Source: three-view drawing plus pictorial views. Frame: mm from the lowest corner of the part. A direction names the side the tool comes from. Give positions to 0.01 mm unless a question says otherwise; leave off trailing zeros. Loops run counter-clockwise (first coordinate to the right, second up) from the corner with the lowest first, then second, coordinate; pieces in that order, holes last.
1. Section C-C, the plane y = 55.5. Output: boundary loops of the cut face in (x, z), then the cut area to 4 significant figures.
2. Section A-A, the plane y = 189. Output: boundary loops of the cut face in (x, z).
3. Material intervals for line 1 along X through (y, z) = (201.75, 40); line 2 along X through (y, z) = (212, 40); line 3 along Z through (x, y) = (155, 203), sorted ascending.
4. Section D-D, the plane z = 71. Output: boundary loops of the cut face in (x, y).
5. Access query for the marked faces 3 and 4. Directions: +Z, -Z, +X, -X, +Y, -Y. A direction counts if a zero-diameter tool reaches every point of the face in a straight line with its end or side. Return the directions, or none.
6. Draft query along X for the marked faces 1 and 2. Return one class per face: +X half, -X half, draft (parallel to the pull), parting line (faces both ways), or undercut.
7. First-contact query: P1, Ø10, axis at x = 212, z = 43, coming from the -Y side; P2, Ø3, axis at x = 108.5, z = 21.5, coming from the -Y side (1 decimal); P3, Ø15, axis at x = 353.5, y = 192, coming from the +Z side; P4, Ø4.5, axis at x = 275, z = 40, coming from the -Y side. Flat tips, straight axial feed; report the tip coordinate or a pass-through.
8. Section B-B, the plane x = 411. Output: boundary loops of the cut face in (y, z).
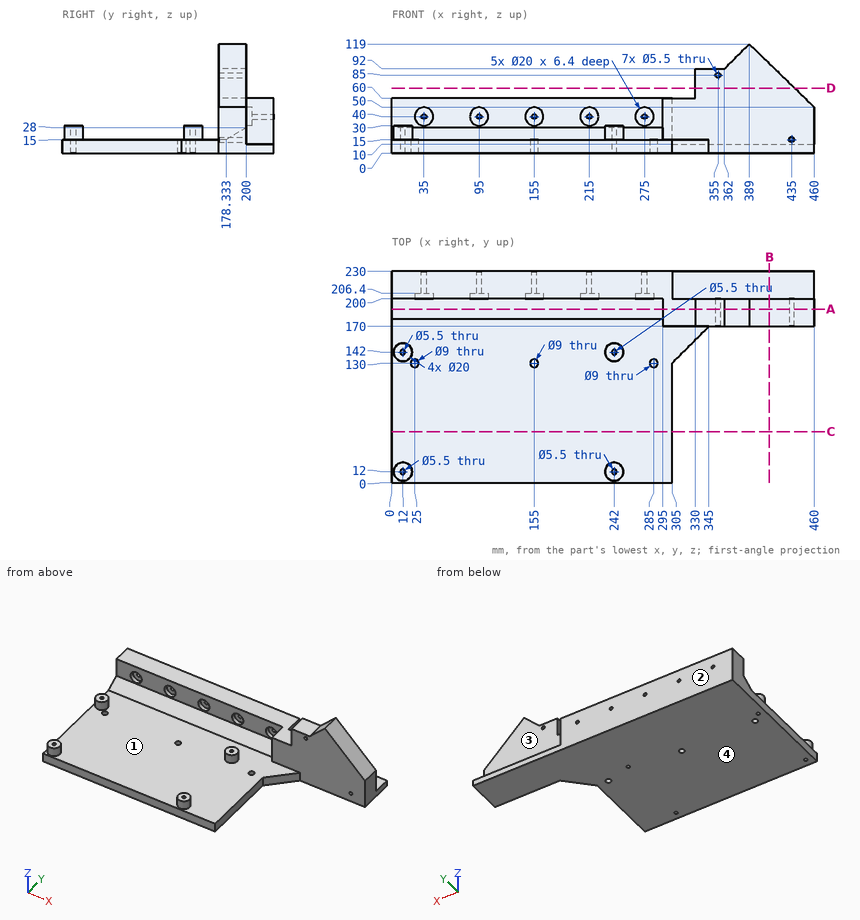
Answers below:
1. outline: (0, 0) - (305, 0) - (305, 15) - (0, 15) - close
1. area: 4,575 mm2
2. outline: (0, 0) - (460, 0) - (460, 50) - (389, 119) - (362, 92) - (330, 92) - (330, 60) - (295, 60) - (295, 21.4) - (0, 21.4) - close; hole circle Ø5.5 at (355, 85); hole circle Ø5.5 at (435, 15)
3. line 1: x = 0 to 25, 45 to 85, 105 to 145, 165 to 205, 225 to 265, 285 to 305
3. line 2: x = 0 to 32.25, 37.75 to 92.25, 97.75 to 152.25, 157.75 to 212.25, 217.75 to 272.25, 277.75 to 305
3. line 3: z = 0 to 30, 50 to 60
4. outline: (330, 170) - (438.39, 170) - (438.39, 200) - (330, 200) - close
5. face 3: +Z, +X, +Y
5. face 4: -Z, +X, -X, +Y, -Y
6. face 1: undercut
6. face 2: draft
7. P1: stops at y = 206.4
7. P2: stops at y = 186.7
7. P3: stops at z = 92
7. P4: passes through
8. outline: (170, 0) - (230, 0) - (230, 10) - (200, 10) - (200, 97.62) - (170, 97.62) - close
